Input: part model. Units: mm. Frame: model coordinates. A direction names the side the tool comes from. Give positions to 0.01 mm unless a question says otherwise; leave off trailing zeros. Order: outer loops, then holes, each group sorted by start corner. A loop starts at its lowest first (then second) coordinate and runs counter-clockwise, first axis right, second up. Notation, with made-up numbers: M 21,88 L 46,88 A11 ccw 46,102 Z; hole C 53,72.5 d5. An arc over 180 degrees is marked long. Use a Markdown table: item, result.
from build123d import *

# Parameters (mm, degrees)
F0_W      = 107.4943505228
F0_H      = 48.250304535
F1_DEPTH  = 10
F2_W      = 37.8673281521
F2_H      = 42.4480531365
F3_DEPTH  = 3
F4_W      = 10.9937405214
F4_H      = 8.8560692966
F5_DEPTH  = 2
F6_W      = 10.9937405214
F6_H      = 8.8560692966
F7_DEPTH  = 2
F8_W      = 10.6883589178
F8_H      = 8.5506872274
F9_DEPTH  = 2
F10_W     = 10.382976383
F10_H     = 8.5506876931
F11_DEPTH = 2
F12_W     = 10.0775957108
F12_H     = 9.1614499688
F13_DEPTH = 2
F14_W     = 10.0775957108
F14_H     = 8.5506867617
F15_DEPTH = 2
F16_W     = 10.6883570552
F16_H     = 8.8560683653
F17_DEPTH = 2
F18_W     = 10.382976383
F18_H     = 9.1614499688
F19_DEPTH = 2
F20_W     = 10.382976383
F20_H     = 8.2453051582
F21_DEPTH = 2
F22_R     = 3.048
F23_R     = 3.048
F24_R     = 3.048
F25_R     = 3.048
F26_R     = 3.048
F27_R     = 0.508
F28_W     = 6.444
F28_H     = 12.8260310739
F29_DEPTH = 7
F30_W     = 11.6044990718
F30_H     = 3.461962243
F31_DEPTH = 2
F32_W     = 9.4668287784
F32_H     = 3.461962243
F33_DEPTH = 2
F34_W     = 4.2035634727
F34_H     = 9.1614509001
F35_DEPTH = 1.5


with BuildPart() as f1:
    # F0 (on Front) → F1 (new body)
    with BuildSketch(Plane.XZ):
        with Locations((3.3591967076, 3.0538169667)):
            Rectangle(F0_W, F0_H)
    extrude(amount=-F1_DEPTH)

    # F2 (on face) → F3 (cut)
    with BuildSketch(Plane.XZ):
        with Locations((35.1188937202, 3.2065073028)):
            Rectangle(F2_W, F2_H)
    extrude(amount=-F3_DEPTH, mode=Mode.SUBTRACT)

    # F4 (on face) → F5 (join)
    with BuildSketch(Plane.XZ):
        with Locations((-5.4968702607, 19.0863553435)):
            Rectangle(F4_W, F4_H)
    extrude(amount=F5_DEPTH)

    # F6 (on face) → F7 (join)
    with BuildSketch(Plane.XZ):
        with Locations((-5.4968702607, 4.4280346483)):
            Rectangle(F6_W, F6_H)
    extrude(amount=F7_DEPTH)

    # F8 (on face) → F9 (join)
    with BuildSketch(Plane.XZ):
        with Locations((-5.3441794589, -10.688358685)):
            Rectangle(F8_W, F8_H)
    extrude(amount=F9_DEPTH)

    # F10 (on face) → F11 (join)
    with BuildSketch(Plane.XZ):
        with Locations((-21.9874810427, 19.2390461452)):
            Rectangle(F10_W, F10_H)
    extrude(amount=F11_DEPTH)

    # F12 (on face) → F13 (join)
    with BuildSketch(Plane.XZ):
        with Locations((-21.8347907066, 4.5807249844)):
            Rectangle(F12_W, F12_H)
    extrude(amount=F13_DEPTH)

    # F14 (on face) → F15 (join)
    with BuildSketch(Plane.XZ):
        with Locations((-21.5294081718, -10.0775957108)):
            Rectangle(F14_W, F14_H)
    extrude(amount=F15_DEPTH)

    # F16 (on face) → F17 (join)
    with BuildSketch(Plane.XZ):
        with Locations((-37.714637816, 19.3917364813)):
            Rectangle(F16_W, F16_H)
    extrude(amount=F17_DEPTH)

    # F18 (on face) → F19 (join)
    with BuildSketch(Plane.XZ):
        with Locations((-37.8673281521, 4.5807249844)):
            Rectangle(F18_W, F18_H)
    extrude(amount=F19_DEPTH)

    # F20 (on face) → F21 (join)
    with BuildSketch(Plane.XZ):
        with Locations((-37.8673281521, -9.924904909)):
            Rectangle(F20_W, F20_H)
    extrude(amount=F21_DEPTH)

    # F22
    f22_edges = [f1.edges().sort_by_distance(p)[0] for p in [
        (-50.387979, 5, -21.071335),
    ]]
    fillet(f22_edges, radius=F22_R)

    # F23
    f23_edges = [f1.edges().sort_by_distance(p)[0] for p in [
        (57.106372, 5, -21.071335),
    ]]
    fillet(f23_edges, radius=F23_R)

    # F24
    f24_edges = [f1.edges().sort_by_distance(p)[0] for p in [
        (57.106372, 5, 27.178969),
    ]]
    fillet(f24_edges, radius=F24_R)

    # F25
    f25_edges = [f1.edges().sort_by_distance(p)[0] for p in [
        (-50.387979, 5, 27.178969),
    ]]
    fillet(f25_edges, radius=F25_R)

    # F26
    f26_edges = [f1.edges().sort_by_distance(p)[0] for p in [
        (3.359197, 10, 27.178969),
    ]]
    fillet(f26_edges, radius=F26_R)

    # F27
    f27_edges = [f1.edges().sort_by_distance(p)[0] for p in [
        (3.359197, 0, 27.178969),
    ]]
    fillet(f27_edges, radius=F27_R)

    # F28 (on face) → F29 (cut)
    with BuildSketch(Plane(origin=(-50.3879785538, 0, 0), x_dir=(0, -1, 0), z_dir=(-1, 0, 0))):
        with Locations((-3.73, 3.0538169667)):
            Rectangle(F28_W, F28_H)
    extrude(amount=-F29_DEPTH, mode=Mode.SUBTRACT)

    # F30 (on face) → F31 (join)
    with BuildSketch(Plane(origin=(0, 0, -21.0713353008), x_dir=(1, 0, 0), z_dir=(0, 0, -1))):
        with Locations((43.0588182062, -2.2389811215)):
            Rectangle(F30_W, F30_H)
    extrude(amount=F31_DEPTH)

    # F32 (on face) → F33 (join)
    with BuildSketch(Plane(origin=(0, 0, -21.0713353008), x_dir=(1, 0, 0), z_dir=(0, 0, -1))):
        with Locations((29.1639482602, -2.2389811215)):
            Rectangle(F32_W, F32_H)
    extrude(amount=F33_DEPTH)

    # F34 (on face) → F35 (join)
    with BuildSketch(Plane.YZ.offset(57.106371969)):
        with Locations((4.8502182637, -8.8560688309)):
            Rectangle(F34_W, F34_H)
    extrude(amount=F35_DEPTH)


solid = f1.part
1) First-contact query: pin 1 Ø1.6 at (y, z) = (-1, 4.5) entering from +X; pin 2 Ø11.5 at (x, z) = (29.5, 13) entering from -Y; pin 3 Ø1 at (x, y) = (-8, -1) entering from -Z. Flat tips, straight axial feed; report the tip coordinate or a pass-through.
Response values:
| item | result |
|---|---|
| pin 1 | stops at x = 0 |
| pin 2 | stops at y = 3 |
| pin 3 | stops at z = -14.96 |
2) Cut plane A-A on y = 1.5. Return loops of the section in (x, z), and give its area (3 significant figures).
Response values:
| item | result |
|---|---|
| outline | M -50.39,-18.02 A3.05 ccw -47.34,-21.07 L 24.43,-21.07 L 24.43,-23.07 L 33.9,-23.07 L 33.9,-21.07 L 37.26,-21.07 L 37.26,-23.07 L 48.86,-23.07 L 48.86,-21.07 L 54.06,-21.07 A3.05 ccw 57.11,-18.02 L 57.11,24.13 A3.05 ccw 54.06,27.18 L -47.34,27.18 A3.05 ccw -50.39,24.13 L -50.39,9.47 L -43.39,9.47 L -43.39,-3.36 L -50.39,-3.36 Z; hole M 16.19,-18.02 L 54.05,-18.02 L 54.05,24.43 L 16.19,24.43 Z |
| area | 3,520 mm² |
3) Material intervals for line 1 (Z direction, x = -10, y = -0.5); line 2 (X direction, y = -1, z = 0.5); line 3 (X direction, y = 1.75, z = 21), sorted ascending. Write a range as from..to.
Response values:
| item | result |
|---|---|
| line 1 | z = -14.96..-6.41, 0..8.86, 14.66..23.51 |
| line 2 | x = -43.06..-32.68, -26.87..-16.8, -10.99..0 |
| line 3 | x = -50.39..16.19, 54.05..57.11 |
4) Mould query, pull axis X, two halves, no side actions, for faces 1 (the face through (-43.059, -1, 5)), 2 (the face through (-16.796, -1, 19)), 3 (the face through (29, 3.97, -22)), 4 (the face through (-16.796, -1, 5)). Classes: released by +X, released by -X, zero draft, split by the parting line, or undercut.
Response values:
| item | result |
|---|---|
| face 1 | released by -X |
| face 2 | undercut |
| face 3 | zero draft |
| face 4 | undercut |
5) Cut plane B-B on x = 6. Return loops of the section in (y, z), and give its area (3 significant figures).
Response values:
| item | result |
|---|---|
| outline | M 0,-20.56 A0.51 ccw 0.51,-21.07 L 6.95,-21.07 A3.05 ccw 10,-18.02 L 10,24.13 A3.05 ccw 6.95,27.18 L 0.51,27.18 A0.51 ccw 0,26.67 Z |
| area | 478 mm² |
6) Cut plane C-C on z = 3.5. Return loops of the section in (x, y), and give its area (3 significant figures).
Response values:
| item | result |
|---|---|
| outline | M -50.39,0.51 A0.51 ccw -49.88,0 L -43.06,0 L -43.06,-2 L -32.68,-2 L -32.68,0 L -26.87,0 L -26.87,-2 L -16.8,-2 L -16.8,0 L -10.99,0 L -10.99,-2 L 0,-2 L 0,0 L 16.19,0 L 16.19,3 L 54.05,3 L 54.05,0 L 56.6,0 A0.51 ccw 57.11,0.51 L 57.11,6.95 A3.05 ccw 54.06,10 L -47.34,10 A3.05 ccw -50.39,6.95 L -43.39,6.95 L -43.39,0.51 Z |
| area | 975 mm² |
7) Cut plane D-D on x = -23. Return loops of the section in (y, z), and give its area (3 significant figures).
Response values:
| item | result |
|---|---|
| outline | M -2,-14.35 L 0,-14.35 L 0,-20.56 A0.51 ccw 0.51,-21.07 L 6.95,-21.07 A3.05 ccw 10,-18.02 L 10,24.13 A3.05 ccw 6.95,27.18 L 0.51,27.18 A0.51 ccw 0,26.67 L 0,23.51 L -2,23.51 L -2,14.96 L 0,14.96 L 0,9.16 L -2,9.16 L -2,0 L 0,0 L 0,-5.8 L -2,-5.8 Z |
| area | 531 mm² |
8) Reachability of faces 5 (the face through (-5, -1, -14.964)), 6 (the face through (-10.994, -1, 19)), 7 (the face through (-38, -1, 9.161)), 8 (the face through (-6, -1, 23.514)), 9 (the face through (43, 3.97, -22)) from +Z, -Z, +X, -X, +Y, -Y: full face, straight path, thin tool, end or side. Return the list, or none.
Response values:
| item | result |
|---|---|
| face 5 | -Z, +X, -X, -Y |
| face 6 | +Z, -Z, -Y |
| face 7 | +X, -X, -Y |
| face 8 | +Z, +X, -Y |
| face 9 | -Z, +X, -X, +Y |
